Job drawing, mm, ordinate dimensions from the low corner. One solid piece. Coordinates: 2 decimals unless noted, no trailing zeros. Order: outer loops, then holes, each group sorted by start corner. A loop starts at its lowest first (then second) coordinate and runs counter-clockwise, first axis right, second up. Notation, with made-up numbers: M 52,52 L 88,52 A23 ccw 88,76 Z; hole C 38,42.25 d9. An arc over 180 degrees is marked long. Write item = value, one per line. Start each with the question number.
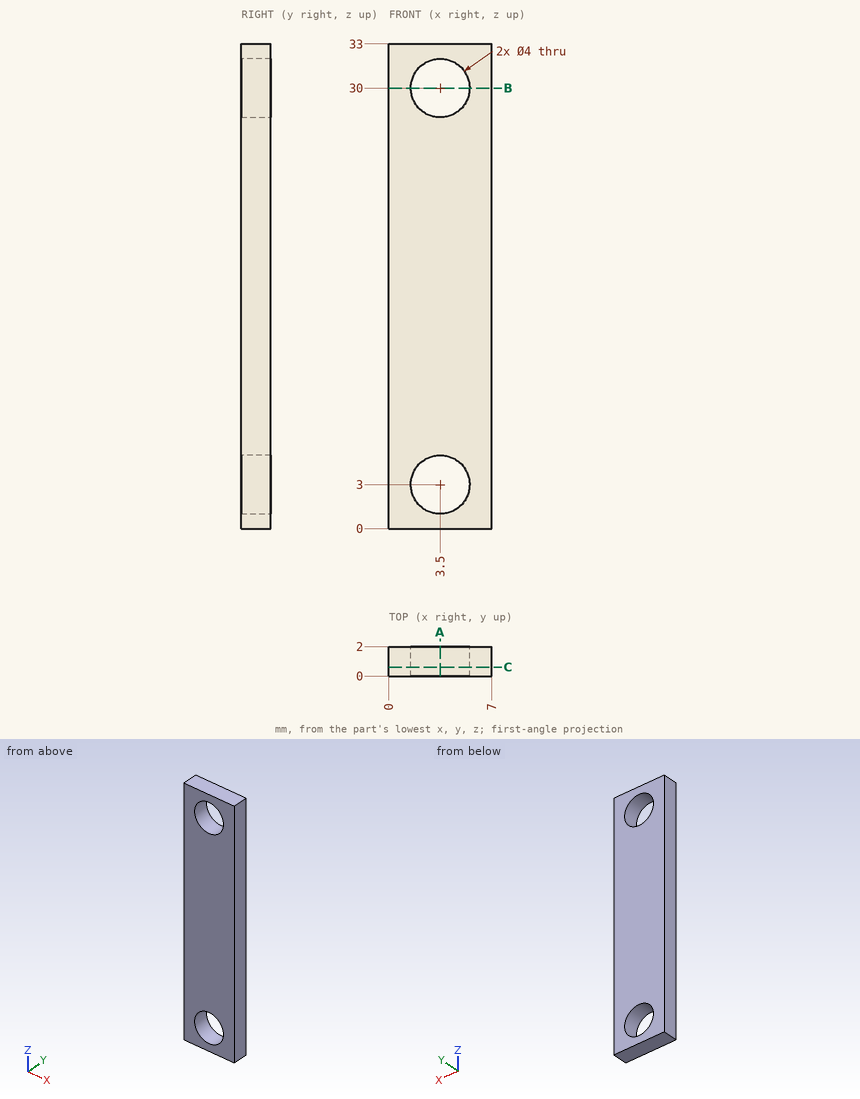
1. Slice it at B-B (z = 30). Write the cut outline in (x, y).
2. Slice it at A-A (x = 3.5). Write the cut outline in (y, z), plus the area to 3 significant figures.
3. Probe L1, parallel to X at y = 1.1, z = 30; L2, parallel to Z at x = 3, y = 0.8; L3, parallel to Z at x = 5, y = 0.8. List the from-to ranges inside material, lowest first.
4. Slice it at C-C (y = 0.6). Write the cut outline in (x, z).
Calculated:
q1.outline = M 0,0 L 1.5,0 L 1.5,2 L 0,2 Z; M 5.5,0 L 7,0 L 7,2 L 5.5,2 Z
q2.outline = M 0,0 L 2,0 L 2,1 L 0,1 Z; M 0,5 L 2,5 L 2,28 L 0,28 Z; M 0,32 L 2,32 L 2,33 L 0,33 Z
q2.area = 50.0 mm²
q3.L1 = 0 to 1.5, 5.5 to 7
q3.L2 = 0 to 1.06, 4.94 to 28.06, 31.94 to 33
q3.L3 = 0 to 1.68, 4.32 to 28.68, 31.32 to 33
q4.outline = M 0,0 L 7,0 L 7,33 L 0,33 Z; hole C 3.5,3 d4; hole C 3.5,30 d4
